Here's how the part is built. I have some questions about the finished solid (model axes, mm). A direction names the side the tool comes from. Coordinates: 2 decimals unless noted, no trailing zeros. Write each loop counter-clockwise with the first axis right and the second up, starting at its lowest first coordinate (ties: lowest second). Pieces come first, ordered by that corner, then holes. Notation, with made-up numbers: M 1.25,-29 L 32.25,-29 A24 cw 32.25,3 Z; hole C 7,88.25 d10. An arc over 180 degrees is marked long. Use a Markdown table: item, result.
```python
from build123d import *

# Parameters (mm, degrees)
SKETCH1_W           = 60
SKETCH1_H           = 50
BOSS_EXTRUDE1_DEPTH = 3
SKETCH2_W           = 10
SKETCH2_H           = 3
CUT_EXTRUDE1_DEPTH  = 3
SKETCH3_R           = 1
CUT_EXTRUDE2_DEPTH  = 10
CAVITY3_START       = -25
CAVITY3_OUTLINE_W   = 3
CAVITY3_OUTLINE_H   = 3
CAVITY3_DEPTH       = 10
CAVITY3_START_2     = -5
CAVITY3_2_OUTLINE_W = 3
CAVITY3_2_OUTLINE_H = 3
CAVITY3_2_DEPTH     = 10
CAVITY3_START_3     = 15
CAVITY3_3_OUTLINE_W = 3
CAVITY3_3_OUTLINE_H = 3
CAVITY3_3_DEPTH     = 7


# Read off the part's stored shape, not the designer's step: Cavity3
with BuildPart() as part:
    # Sketch1 → Boss-Extrude1 (new body)
    with BuildSketch(Plane.XY):
        Rectangle(SKETCH1_W, SKETCH1_H)
    extrude(amount=BOSS_EXTRUDE1_DEPTH)

    # Sketch2 → Cut-Extrude1 (cut)
    with BuildSketch(Plane.XY.offset(3)):
        with Locations((-15, 23.5)):
            Rectangle(SKETCH2_W, SKETCH2_H)
        with Locations((15, 23.5)):
            Rectangle(SKETCH2_W, SKETCH2_H)
    extrude(amount=-CUT_EXTRUDE1_DEPTH, mode=Mode.SUBTRACT)

    # Sketch3 → Cut-Extrude2 (cut)
    with BuildSketch(Plane.XY.offset(3)):
        with Locations((0, 3)):
            Circle(SKETCH3_R)
        with Locations((3, 0)):
            Circle(SKETCH3_R)
        with Locations((0, -3)):
            Circle(SKETCH3_R)
        with Locations((-3, 0)):
            Circle(SKETCH3_R)
    extrude(amount=-CUT_EXTRUDE2_DEPTH, mode=Mode.SUBTRACT)

    # Cavity3 outline → Cavity3 (cut)
    with BuildSketch(Plane(origin=(0, 0, 0), x_dir=(1, 0, 0), z_dir=(0, 1, 0)).offset(CAVITY3_START)):
        with Locations((28.5, -1.5)):
            Rectangle(CAVITY3_OUTLINE_W, CAVITY3_OUTLINE_H)
        with Locations((-28.5, -1.5)):
            Rectangle(CAVITY3_OUTLINE_W, CAVITY3_OUTLINE_H)
    extrude(amount=CAVITY3_DEPTH, mode=Mode.SUBTRACT)

    # Cavity3 2 outline → Cavity3 2 (cut)
    with BuildSketch(Plane(origin=(0, 0, 0), x_dir=(1, 0, 0), z_dir=(0, 1, 0)).offset(CAVITY3_START_2)):
        with Locations((28.5, -1.5)):
            Rectangle(CAVITY3_2_OUTLINE_W, CAVITY3_2_OUTLINE_H)
        with Locations((-28.5, -1.5)):
            Rectangle(CAVITY3_2_OUTLINE_W, CAVITY3_2_OUTLINE_H)
    extrude(amount=CAVITY3_2_DEPTH, mode=Mode.SUBTRACT)

    # Cavity3 3 outline → Cavity3 3 (cut)
    with BuildSketch(Plane(origin=(0, 0, 0), x_dir=(1, 0, 0), z_dir=(0, 1, 0)).offset(CAVITY3_START_3)):
        with Locations((28.5, -1.5)):
            Rectangle(CAVITY3_3_OUTLINE_W, CAVITY3_3_OUTLINE_H)
        with Locations((-28.5, -1.5)):
            Rectangle(CAVITY3_3_OUTLINE_W, CAVITY3_3_OUTLINE_H)
    extrude(amount=CAVITY3_3_DEPTH, mode=Mode.SUBTRACT)


solid = part.part
```
1. We'd pull the mould along X, two halves only. Please class faces 1 (the face through (20, 23, 2)), 2 (the face through (-27, 18, 2)), 3 (the face through (0, 0, 0)), 4 (the face through (27, 18, 2)): +X half, -X half, draft (parallel to the pull), parting line (faces both ways), or undercut.
Answers follow:
| item | result |
|---|---|
| face 1 | undercut |
| face 2 | -X half |
| face 3 | draft |
| face 4 | +X half |
2. Suppose I cut it at C-C on z = 0.45. State how many separate pieces and enclosed holes the cut face has, and give its area (3 significant figures).
Answers follow:
| item | result |
|---|---|
| separate pieces | 1 |
| enclosed holes | 4 |
| area | 2,770 mm2 |
3. Suppose I cut it at D-D on x = -16. Write out the boundary of the cut face in (y, z), and give its area (3 significant figures).
Answers follow:
| item | result |
|---|---|
| outline | M -25,0 L 22,0 L 22,3 L -25,3 Z |
| area | 141 mm2 |
4. Suppose I cut it at A-A on y = 0. Write out the boundary of the cut face in (x, z).
Answers follow:
| item | result |
|---|---|
| outline | M -27,0 L -4,0 L -4,3 L -27,3 Z; M -2,0 L 2,0 L 2,3 L -2,3 Z; M 4,0 L 27,0 L 27,3 L 4,3 Z |
5. Suppose I cut it at B-B on x = 3. Write out the boundary of the cut face in (y, z), and give its area (3 significant figures).
Answers follow:
| item | result |
|---|---|
| outline | M -25,0 L -1,0 L -1,3 L -25,3 Z; M 1,0 L 25,0 L 25,3 L 1,3 Z |
| area | 144 mm2 |
6. I need wall thicknesses on probe 1 along Y at (x, z) = (0, 1.95); probe 2 along Y at (x, z) = (-3, 1.3); probe 3 along X at (y, z) = (1.5, 1.6). Which ranges of each line are inside material? Lowest first, please.
Answers follow:
| item | result |
|---|---|
| probe 1 | y = -25 to -4, -2 to 2, 4 to 25 |
| probe 2 | y = -25 to -1, 1 to 25 |
| probe 3 | x = -27 to 27 |
7. Which directions (+Z, -Z, +X, -X, +Y, -Y) give clear straight access to the entire face, cutting with the end or side of a thin tool? Please do faces 5 (the face through (27, 0, 2)), 6 (the face through (15, 22, 2)), 7 (the face through (-29, 15, 1)).
Answers follow:
| item | result |
|---|---|
| face 5 | +Z, -Z, +X |
| face 6 | +Z, -Z, +Y |
| face 7 | +Z, -Z, -X |
8. Will these pins go through, and if not, where does the flat tip stop? pin 1 Ø0.9 at (y, z) = (-18.5, 1) entering from -X; pin 2 Ø4 at (x, y) = (16.5, -16.5) entering from -Z; pin 3 Ø1.5 at (x, z) = (28.5, 1) entering from -Y; pin 4 Ø1.2 at (x, y) = (0, 3) entering from -Z.
Answers follow:
| item | result |
|---|---|
| pin 1 | stops at x = -27 |
| pin 2 | stops at z = 0 |
| pin 3 | stops at y = -15 |
| pin 4 | passes through |
